Could you check a few things on this drawing? It's one solid part, dimensions in mm from its lowest x, y, z. A direction names the side the tool comes from. Coordinates: 2 decimals unless noted, no trailing zeros. Loops run counter-clockwise (first coordinate to the right, second up) from the corner with the lowest first, then second, coordinate; pieces in that order, holes last. Notation, with made-up numbers: M 85,5.25 L 126,5.25 A19 cw 126,14.25 Z; hole C 75,53 d3. An arc over 180 degrees is marked long. Answer as a JSON object with one key per item and string values. Group by question number.
Item 1: Suppose I cut it at A-A (z = 6). Count the separate pieces of the cut face and the enclosed holes in it.
Item 2: Which directions (+Z, -Z, +X, -X, +Y, -Y) give clear straight access to the entire face, cutting with the end or side of a thin tool? Please do the marked faces 4 and 5.
Item 3: If I drill on line 1 (X direction, y = 1.5, z = 4.25) (1 decimal); line 2 (Z direction, x = 5, y = 4.25); line 3 (X direction, y = 3.25, z = 6.5) (1 decimal), over which ranges is the centre line in solid material (lowest first)?
Item 4: I'm going to push flat-ended pins straight in: pin 1 Ø1.5 at (x, z) = (4, 6.5) entering from +Y; pin 2 Ø4.5 at (x, z) = (31.5, 5.5) entering from +Y; pin 3 Ø6 at (y, z) = (6, 10) entering from +X. Where does each tip first touch, or does it pass through?
Item 5: We'd pull the mould along Z, two halves only. Please class the marked faces 1, 2 and 3: +Z half, -Z half, draft (parallel to the pull), parting line (faces both ways), or undercut.
Item 6: Suppose I cut it at D-D (y = 13.5). Write out the boundary of the cut face in (x, z), then the cut area to 3 significant figures.
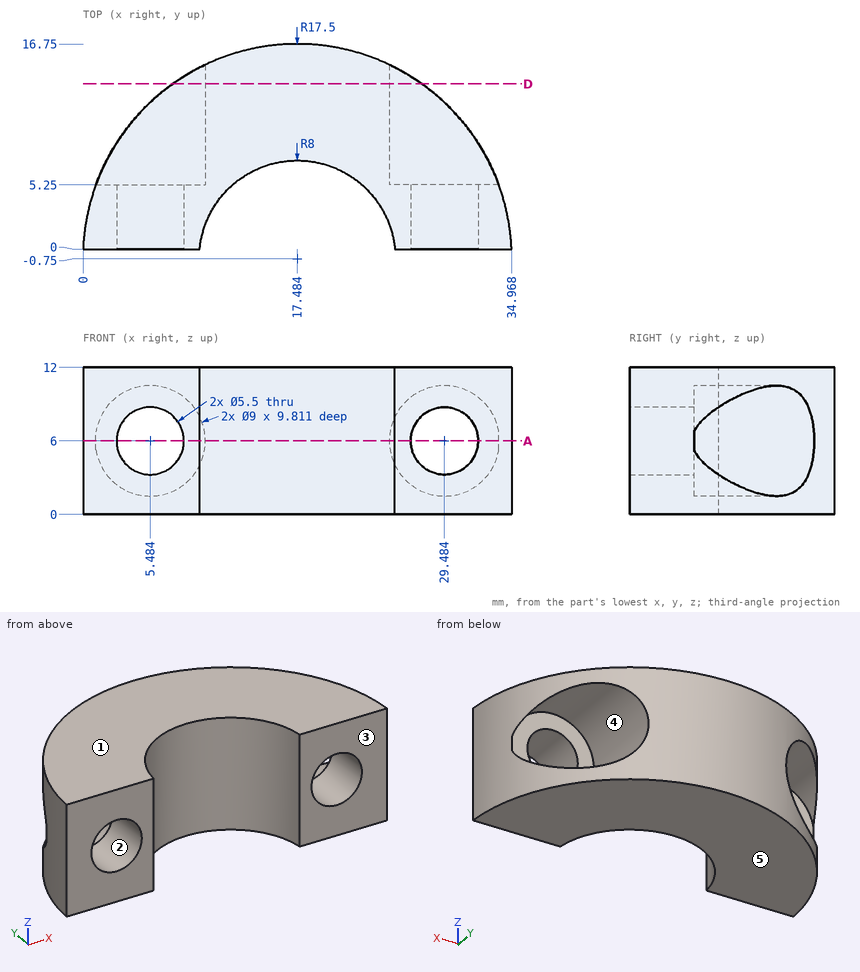
From the geometry:
{
 "1": {"separate pieces": "3", "enclosed holes": "0"},
 "2": {"face 4": "+Y", "face 5": "-Z, +X, -X, +Y, -Y"},
 "3": {"line 1": "0.1 to 3.4, 7.6 to 9.8, 25.2 to 27.4, 31.6 to 34.8", "line 2": "0 to 3.29, 8.71 to 12", "line 3": "0.4 to 2.8, 8.2 to 10.6, 24.4 to 26.8, 32.2 to 34.5"},
 "4": {"pin 1": "through", "pin 2": "y = 5.25", "pin 3": "x = 34.58"},
 "5": {"face 1": "+Z half", "face 2": "undercut", "face 3": "draft"},
 "6": {"outline": "M 7.33,0 L 27.64,0 L 27.64,1.89 A4.5 cw 27.64,10.11 L 27.64,12 L 7.33,12 L 7.33,10.11 A4.5 cw 7.33,1.89 Z", "area": "212 mm2"}
}
